from build123d import *

# Parameters (mm, degrees)
F1_DEPTH = 25.4
F2_R     = 6.35
F3_DEPTH = 6.35
F4_R     = 3.937
F5_DEPTH = 25.4
F7_DEPTH = 52.7686600304
F9_DEPTH = 25.4


with BuildPart() as f1:
    # F0 (on Front) → F1 (new body, symmetric)
    with BuildSketch(Plane.XZ):
        Polygon((-85.852, 12.7), (-85.852, 0), (0, 0), (45.8512699094, -45.8512699094), (54.8315260304, -36.8710137883), (17.5184486888, 0.4420635534), (5.2605122421, 12.7), align=None)
        Polygon((26.4987048099, 9.4223196744), (17.5184486888, 0.4420635534), (54.8315260304, -36.8710137883), (63.8117821515, -27.8907576672), align=None)
    extrude(amount=F1_DEPTH, both=True)

    # F2 (on face) → F3 (cut)
    with BuildSketch(Plane(origin=(0, 0, 0), x_dir=(1, 0, 0), z_dir=(0, 0, -1))):
        with Locations((-70.104, 12.7)):
            Circle(F2_R)
        with Locations((-16.256, 12.7)):
            Circle(F2_R)
        with Locations((-16.256, -12.7)):
            Circle(F2_R)
        with Locations((-70.104, -12.7)):
            Circle(F2_R)
    extrude(amount=-F3_DEPTH, mode=Mode.SUBTRACT)

    # F4 (on face) → F5 (cut)
    with BuildSketch(Plane(origin=(0, 0, 0), x_dir=(1, 0, 0), z_dir=(0, 0, -1))):
        with Locations((-16.256, -12.7)):
            Circle(F4_R)
        with Locations((-16.256, 12.7)):
            Circle(F4_R)
        with Locations((-70.104, 12.7)):
            Circle(F4_R)
        with Locations((-70.104, -12.7)):
            Circle(F4_R)
    extrude(amount=-F5_DEPTH, mode=Mode.SUBTRACT)

    # F6 (on face) → F7 (cut, through all)
    with BuildSketch(Plane(origin=(45.8512699094, 0, -45.8512699094), x_dir=(0, 1, 0), z_dir=(0.7071067812, 0, -0.7071067812))):
        Polygon((9.652, 25.4), (-9.652, 25.4), (-9.652, 19.304), (-15.748, 19.304), (-15.748, 12.7), (15.748, 12.7), (15.748, 19.304), (9.652, 19.304), align=None)
    extrude(amount=-F7_DEPTH, mode=Mode.SUBTRACT)

    # F8 (on face) → F9 (cut, through all)
    with BuildSketch(Plane(origin=(17.9605122421, 0, 17.9605122421), x_dir=(0, 1, 0), z_dir=(0.7071067812, 0, 0.7071067812))):
        with BuildLine():
            ThreePointArc((-9.652, -63.8151974917), (-17.7699630745, -61.5408606446), (-25.4, -57.9552687705))
            Line((-25.4, -57.9552687705), (-25.4, -64.8434877579))
            Line((-25.4, -64.8434877579), (-9.652, -64.8434877579))
            Line((-9.652, -64.8434877579), (-9.652, -63.8151974917))
        make_face()
        with BuildLine():
            ThreePointArc((25.4, -57.89321661), (8.408914861, -64.0203496104), (-9.652, -63.8151974917))
            Line((-9.652, -63.8151974917), (-9.652, -64.8434877579))
            Line((-9.652, -64.8434877579), (1.0093030718, -64.8434877579))
            Line((1.0093030718, -64.8434877579), (25.4, -64.8434877579))
            Line((25.4, -64.8434877579), (25.4, -57.89321661))
        make_face()
    extrude(amount=-F9_DEPTH, mode=Mode.SUBTRACT)


solid = f1.part
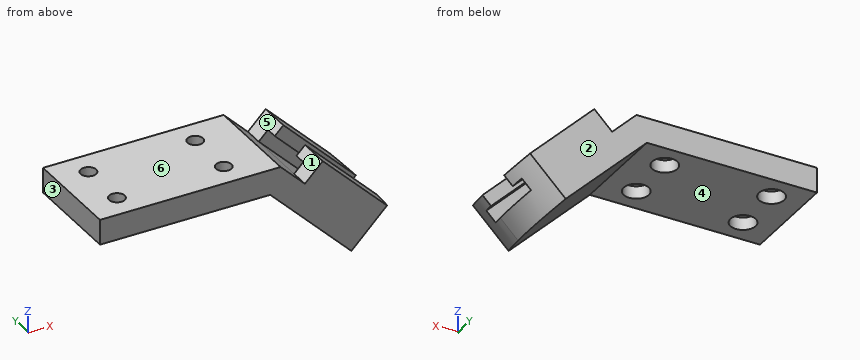
Source: CAD feature listing. Evaluate the final solid. Frame: model axes, mm. Face numbers are marked on the shaded views. A direction names the side the tool comes from. Coordinates: 2 decimals unless noted, no trailing zeros. Loops run counter-clockwise (first coordinate to the right, second up) from the corner with the lowest first, then second, coordinate; pieces in that order, holes last. Notation, with made-up numbers: M 17.25,45.25 L 51.25,45.25 A7 cw 51.25,51.25 Z; hole C 36.25,-15 d3. An arc over 180 degrees is marked long. Answer in a Markdown table with one row per item.
Q1. Section D-D on y = 0.5. Return the cut outline in (x, z), plus the area to 3 significant figures.
Answers below:
| item | result |
|---|---|
| outline | M -85.85,0 L 0,0 L 45.77,-45.77 L 54.75,-36.79 L 5.26,12.7 L -85.85,12.7 Z |
| area | 1,980 mm^2 |
Q2. First-contact query: pin 1 (10 mm diameter, centred on x = -71.5, y = -11, fed in from -Z); pin 2 (9 mm diameter, centred on x = -16.256, y = 12.7, fed in from -Z); pin 3 (4 mm diameter, centred on y = 7.5, z = -26.5, fed in from -X). Flat tips, straight axial feed; report the tip coordinate or a pass-through.
Answers below:
| item | result |
|---|---|
| pin 1 | stops at z = 0 |
| pin 2 | stops at z = 6.35 |
| pin 3 | stops at x = 24.5 |
Q3. Draft query along X for the marked faces 1, 2 and 3. Return one class per face: pulls with the +X half, pulls with the -X half, needs draft (parallel to the pull), parting line crosses it, or undercut.
Answers below:
| item | result |
|---|---|
| face 1 | undercut |
| face 2 | needs draft |
| face 3 | pulls with the -X half |
Q4. Ray query, probe 1 along X at (y, z) = (12.7, 11.5); probe 2 along X at (y, z) = (9, 2.5); probe 3 along X at (y, z) = (-12, 9). Return the intervals inside material, ascending. Write a range as from..to.
Answers below:
| item | result |
|---|---|
| probe 1 | x = -85.85..-74.04, -66.17..-20.19, -12.32..6.46 |
| probe 2 | x = -85.85..-75.26, -64.94..-21.42, -11.1..15.46 |
| probe 3 | x = -85.85..-73.98, -66.23..-20.13, -12.38..8.96, 26.08..26.92 |
Q5. Section A-A on y = -12.7. Return the cut outline in (x, z), plus the area to 3 significant figures.
Answers below:
| item | result |
|---|---|
| outline | M -85.85,0 L -76.45,0 L -76.45,6.35 L -74.04,6.35 L -74.04,12.7 L -85.85,12.7 Z; M -66.17,6.35 L -63.75,6.35 L -63.75,0 L -22.61,0 L -22.61,6.35 L -20.19,6.35 L -20.19,12.7 L -66.17,12.7 Z; M -12.32,6.35 L -9.91,6.35 L -9.91,0 L 0,0 L 44.64,-44.64 L 53.62,-35.66 L 5.26,12.7 L -12.32,12.7 Z; M 22.19,5.11 L 58.29,-30.99 L 62.6,-26.68 L 26.5,9.42 Z |
| area | 2,010 mm^2 |
Q6. Set-up query: the marked faces 4, 5 and 6. Return all of +Z, -Z, +X, -X, +Y, -Y with unobstructed straight access to the full face (end or side cutting, diameter ignored); none if empty.
Answers below:
| item | result |
|---|---|
| face 4 | -Z, -X, +Y, -Y |
| face 5 | +Z, +Y, -Y |
| face 6 | +Z, +X, -X, +Y, -Y |
Q7. Section B-B on z = -17.5. Return the cut outline in (x, y).
Answers below:
| item | result |
|---|---|
| outline | M 17.5,-25.4 L 53.42,-25.4 L 53.42,-9.65 L 44.8,-9.65 L 44.8,-15.75 L 35.46,-15.75 L 35.46,15.75 L 44.8,15.75 L 44.8,9.65 L 53.42,9.65 L 53.42,25.4 L 17.5,25.4 Z |
Q8. Section C-C on x = -51.5. Return the cut outline in (y, z), plus the area to 3 significant figures.
Answers below:
| item | result |
|---|---|
| outline | M -25.4,0 L 25.4,0 L 25.4,12.7 L -25.4,12.7 Z |
| area | 645 mm^2 |
